Verification items for the finished model (mm, model axes). Face numbers are marked on the shaded views. A direction names the side the tool comes from. Give positions to 0.01 mm unless a question says otherwise; leave off trailing zeros. Write each loop counter-clockwise with the first axis right and the second up, starting at its lowest first coordinate (ties: lowest second). Pieces come first, ordered by that corner, then holes. Notation, with made-up numbers: (68.25, -13.5) - (106.25, -13.5) arc R12 ccw to (106.25, -9.5) - close; hole circle Ø4 at (67, 63.5). An arc over 180 degrees is marked (long way). Answer as a JSON object with one key per item and string values. Group by question number.
Item 1: Draft check along Z on the marked faces 3, 4, 5 and 6. Enter one of: +Z half, -Z half, draft (parallel to the pull), parting line (faces both ways), or undercut.
Item 2: Tool access check on the marked faces 1 and 2. Record the directions out of +Z, -Z, +X, -X, +Y, -Y that give a thin tool (end or side, any length) a straight path to the whole face; none if there is none.
Item 3: Sectioned sample at B-B, the plane z = 0. Record the boundary of the cut face in (x, y), and give its area (3 significant figures).
Item 4: Sectioned sample at C-C, the plane y = -1.7. Record the boundary of the cut face in (x, z), and give its area (3 significant figures).
Item 5: Sectioned sample at A-A, the plane x = 0. Record the boundary of the cut face in (y, z) (3 decimals).
Item 6: Scan lines: line 1 along X through (y, z) = (0, 0.5); line 2 along X through (y, z) = (1.95, -1); line 3 along Y through (x, z) = (0, -2.75) (3 decimals). Record each from-to range of solid material in increasing order. Write a range as [from, to].
Item 7: Sectioned sample at D-D, the plane y = 0. Record the boundary of the cut face in (x, z) (3 decimals), and give its area (3 significant figures).
Item 8: Go/stop test with flat-tipped pins: pin 1 (2 mm diameter, centred on x = -6, z = 0, fed in from -Y); pin 2 (2.5 mm diameter, centred on x = 0, y = 0, fed in from -Z); pin 3 (1 mm diameter, centred on x = 5, y = 1.5, fed in from +Z). Record where each tip stops, or that it passes through.
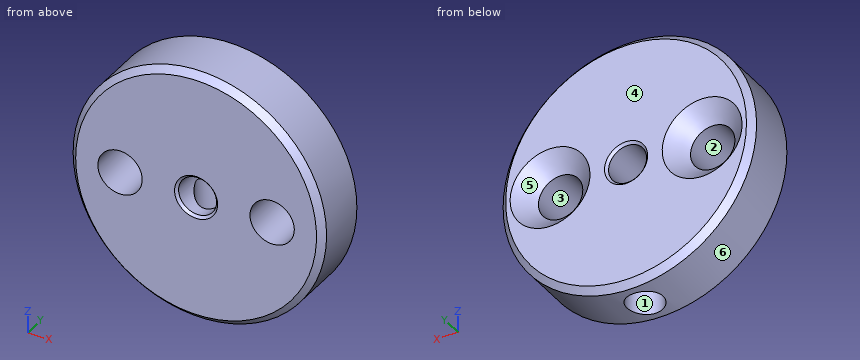
Autodesk Inventor part; units mm, degrees
ref_plane "YZ Plane" through (0, 0, 0) normal (1, 0, 0) x (0, 1, 0)
ref_plane "XZ Plane" through (0, 0, 0) normal (0, 1, 0) x (-1, 0, 0)
ref_plane "XY Plane" through (0, 0, 0) normal (0, 0, 1) x (1, 0, 0)
sketch "Sketch4" plane through (0, 0, 0) normal (0, 1, 0) x (-1, 0, 0)
  circle A0 centre (0, 0) radius 10
extrude "Extrusion2" add sketch "Sketch4" along normal mid plane 5
sketch "Sketch8" plane through (0, 2.5, 0) normal (0, 1, 0) x (1, 0, 0)
  point P0 (0, 0)
  point P1 (-6, 0)
  point P2 (6, 0)
  dimension "d63" = 6
  dimension "d64" = 12
hole "Hole5" at (-6, 2.5, 0) at (6, 2.5, 0) direction (0, -1, 0) diameter 3.5 depth 22.2 countersink diameter 6.3 countersink angle 90
sketch "Sketch9" plane through (0, 2.5, 0) normal (0, 1, 0) x (1, 0, 0)
  line L0 (-1.5, 1.5) -> (1.5, 1.5) construction
  line L1 (1.5, 1.5) -> (1.5, -1.5) construction
  line L2 (1.5, -1.5) -> (-1.5, -1.5) construction
  line L3 (-1.5, -1.5) -> (-1.5, 1.5) construction
  line L4 (-1.5, 1.5) -> (1.5, -1.5) construction
  line L5 (1.5, 1.5) -> (-1.5, -1.5) construction
  circle A0 centre (0, 0) radius 1.5
  dimension "d72" = 3
  dimension "d73" = 3
  dimension "d86" = 3
extrude "Extrusion5" cut sketch "Sketch9" against normal blind 10
sketch "Sketch10" plane through (-1.5, 2.5, 0) normal (0, 0, 1) x (1, 0, 0)
  point P0 (1.5, -2.5)
  point P1 (1.5, -2.5)
hole "Hole6" at (0, 0, 0) direction (0, 0, -1) diameter 2.85 depth 10.4
chamfer "Chamfer1" distance 0.5 angle 45 2 edges at (10, 2.5, 0) (10, -2.5, 0)
chamfer "Chamfer2" distance 0.2 angle 45 2 edges at (-1.5, 2.5, 0) (-1.5, -2.5, 0)
equation "\"d73\" = d72"
properties part number "Wheel Mounting Cap" material "Mild Steel S355 J2"
Geometry check:
{
 "1": {"face 3": "undercut", "face 4": "draft", "face 5": "undercut", "face 6": "parting line"},
 "2": {"face 1": "-Z", "face 2": "+Y, -Y"},
 "3": {"outline": "(-10, -2) - (-9.5, -2.5) - (-7.75, -2.5) - (-7.75, 1.1) - (-9.15, 2.5) - (-9.5, 2.5) - (-10, 2) - close; (-4.25, -2.5) - (-1.7, -2.5) - (-1.5, -2.3) - (-1.5, 2.3) - (-1.7, 2.5) - (-2.85, 2.5) - (-4.25, 1.1) - close; (1.5, -2.3) - (1.7, -2.5) - (4.25, -2.5) - (4.25, 1.1) - (2.85, 2.5) - (1.7, 2.5) - (1.5, 2.3) - close; (7.75, -2.5) - (9.5, -2.5) - (10, -2) - (10, 2) - (9.5, 2.5) - (9.15, 2.5) - (7.75, 1.1) - close", "area": "45.5 mm^2"},
 "4": {"outline": "circle Ø20 at (0, 0); hole circle Ø3.5 at (-6, 0); hole circle Ø3 at (0, 0); hole circle Ø3.5 at (6, 0)", "area": "288 mm^2"},
 "5": {"outline": "(-2.5, -9.5) - (-2, -10) - (-1.425, -10) - (-1.425, -1.5) - (-2.3, -1.5) - (-2.5, -1.7) - close; (-2.5, 1.7) - (-2.3, 1.5) - (2.3, 1.5) - (2.5, 1.7) - (2.5, 9.5) - (2, 10) - (-2, 10) - (-2.5, 9.5) - close; (1.425, -10) - (2, -10) - (2.5, -9.5) - (2.5, -1.7) - (2.3, -1.5) - (1.425, -1.5) - close"},
 "6": {"line 1": "[-9.99, -7.68], [-4.32, -1.41], [1.41, 4.32], [7.68, 9.99]", "line 2": "[-9.95, -8.4], [-3.6, -1.12], [1.12, 3.6], [8.4, 9.95]", "line 3": "[-2.5, -1.425], [1.425, 2.5]"},
 "7": {"outline": "(-1.425, -9.898) - (-1.425, -0.468) arc R1.5 cw (long way) to (1.425, -0.468) - (1.425, -9.898) arc R10 ccw (long way) to start; hole circle Ø3.5 at (-6, 0); hole circle Ø3.5 at (6, 0)", "area": "263 mm^2"},
 "8": {"pin 1": "through", "pin 2": "z = 0.83", "pin 3": "z = 8.93"}
}
